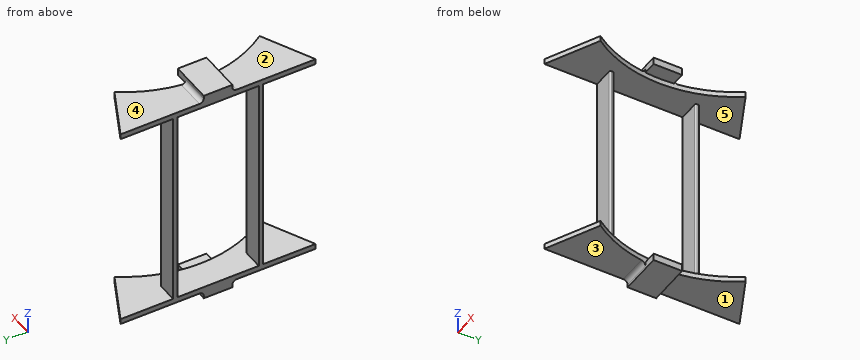
from build123d import *

# Parameters (mm, degrees)
BOSS_EXTRUDE1_DEPTH = 1.875
BOSS_EXTRUDE3_DEPTH = 140
BOSS_EXTRUDE4_DEPTH = 5
FILLET4_R           = 3


with BuildPart() as part:
    # Sketch1 → Boss-Extrude1 (new body, symmetric)
    with BuildSketch(Plane.XY):
        with BuildLine():
            Line((-72.585877034, -50.825178267), (-108.610994186, -68.325178267))
            Line((-108.610994186, -68.325178267), (-108.610994186, 68.325178267))
            Line((-108.610994186, 68.325178267), (-72.585877034, 50.825178267))
            ThreePointArc((-72.585877034, 50.825178267), (-88.610994186, 0), (-72.585877034, -50.825178267))
        make_face()
    boss_extrude1 = extrude(amount=BOSS_EXTRUDE1_DEPTH, both=True)

    # Sketch3 → Boss-Extrude3 (add)
    with BuildSketch(Plane.XY.offset(1.875)):
        with BuildLine():
            Line((-108.610994186, -28.5), (-108.610994186, -31.5))
            Line((-108.610994186, -31.5), (-94.610994186, -31.5))
            ThreePointArc((-94.610994186, -31.5), (-93.903887405, -31.207106781), (-93.610994186, -30.5))
            Line((-93.610994186, -30.5), (-93.610994186, -29.5))
            ThreePointArc((-93.610994186, -29.5), (-93.903887405, -28.792893219), (-94.610994186, -28.5))
            Line((-94.610994186, -28.5), (-108.610994186, -28.5))
        make_face()
    boss_extrude3 = extrude(amount=BOSS_EXTRUDE3_DEPTH)

    # Mirror2: Boss-Extrude3 across plane
    add(boss_extrude3.mirror(Plane.ZX))

    # Mirror7: Boss-Extrude1 across plane
    add(boss_extrude1.mirror(Plane.XY.offset(71.875)))

    # Sketch4 → Boss-Extrude4 (add)
    with BuildSketch(Plane(origin=(0, 0, -1.875), x_dir=(-1, 0, 0), z_dir=(0, 0, -1))):
        Polygon((108.610994186, 0), (108.610994186, 10), (78.610994186, 10), (78.610994186, -10), (108.610994186, -10), align=None)
    boss_extrude4 = extrude(amount=BOSS_EXTRUDE4_DEPTH)

    # Mirror10: Boss-Extrude4 across plane
    add(boss_extrude4.mirror(Plane.XY.offset(71.875)))

    # Fillet4
    fillet4_edges = [part.edges().sort_by_distance(p)[0] for p in [
        (-98.327958095, -10, -1.875),
        (-98.327958095, 10, -1.875),
        (-98.327958095, -10, 145.625),
        (-98.327958095, 10, 145.625),
    ]]
    fillet(fillet4_edges, radius=FILLET4_R)


solid = part.part
For this review, take the finished solid that the model builds, in its own axes (mm). Face numbers are marked on the shaded views. A direction names the side the tool comes from. Give positions to 0.01 mm unless a question says otherwise; leave off trailing zeros. Write each loop counter-clockwise with the first axis right and the second up, starting at its lowest first coordinate (ties: lowest second). Pieces come first, ordered by that corner, then holes. Notation, with made-up numbers: (75.5, 59) -> (125.5, 59) arc R18 cw to (125.5, 88) -> close; hole circle Ø11 at (32, 37.5). An arc over 180 degrees is marked (long way). Use CSV: the item, a comma, the result in double quotes.
Q1. Tool access review of the marked faces 1, 2 and 3: name each direction out of +Z, -Z, +X, -X, +Y, -Y from which nothing blocks a thin tool from reaching the whole face with its end or side.
Conclusion:
face 1,"-Z, +X, -X, +Y"
face 2,"+Z, +X, -X, -Y"
face 3,"-Z, +X, -X, -Y"
Q2. Take a section at D-D, the plane x = -98.5. Write out the cut boundary in (y, z) (3 decimals).
Conclusion:
outline,"(-63.414, -1.875) -> (-13, -1.875) arc R3 cw to (-10, -4.875) -> (-10, -6.875) -> (10, -6.875) -> (10, -4.875) arc R3 cw to (13, -1.875) -> (63.414, -1.875) -> (63.414, 1.875) -> (31.5, 1.875) -> (31.5, 141.875) -> (63.414, 141.875) -> (63.414, 145.625) -> (13, 145.625) arc R3 cw to (10, 148.625) -> (10, 150.625) -> (-10, 150.625) -> (-10, 148.625) arc R3 cw to (-13, 145.625) -> (-63.414, 145.625) -> (-63.414, 141.875) -> (-31.5, 141.875) -> (-31.5, 1.875) -> (-63.414, 1.875) -> close; hole (-28.5, 1.875) -> (28.5, 1.875) -> (28.5, 141.875) -> (-28.5, 141.875) -> close"
Q3. Take a section at A-A, the plane y = 0. Write out the cut boundary in (x, z) (3 decimals), then the cut area to 3 significant figures.
Conclusion:
outline,"(-108.611, -6.875) -> (-78.611, -6.875) -> (-78.611, -1.875) -> (-88.611, -1.875) -> (-88.611, 1.875) -> (-108.611, 1.875) -> close; (-108.611, 141.875) -> (-88.611, 141.875) -> (-88.611, 145.625) -> (-78.611, 145.625) -> (-78.611, 150.625) -> (-108.611, 150.625) -> close"
area,"450 mm2"
Q4. Mouldability with a two-part tool opening along Y and no side actions: class the marked faces 4 and 5 as pulls with the +Y half, pulls with the -Y half, needs draft (parallel to the pull), parting line crosses it, or undercut.
Conclusion:
face 4,"needs draft"
face 5,"undercut"
Q5. To check wall thickness, follow probe 1 along Z at (x, y) = (-95.5, -13.5) (3 decimals); probe 2 along Z at (x, y) = (-103, -2) (3 decimals); probe 3 along Y at (x, z) = (-105.5, 126). State the ranges of each line that lie inside material, in increasing order. Write a range as [from, to].
Conclusion:
probe 1,"[-1.875, 1.875], [141.875, 145.625]"
probe 2,"[-6.875, 1.875], [141.875, 150.625]"
probe 3,"[-31.5, -28.5], [28.5, 31.5]"
Q6. Take a section at B-B, the plane z = 79.5. Write out the cut boundary in (x, y), then the cut area to 3 significant figures.
Conclusion:
outline,"(-108.61, -31.5) -> (-94.61, -31.5) arc R1 ccw to (-93.61, -30.5) -> (-93.61, -29.5) arc R1 ccw to (-94.61, -28.5) -> (-108.61, -28.5) -> close; (-108.61, 28.5) -> (-94.61, 28.5) arc R1 ccw to (-93.61, 29.5) -> (-93.61, 30.5) arc R1 ccw to (-94.61, 31.5) -> (-108.61, 31.5) -> close"
area,"89.1 mm2"
Q7. For P1, Ø8, axis at x = -92.5, z = 110, coming from the -Y side; P2, Ø5, axis at y = -33.5, z = 115, coming from the +X side; P3, Ø5.5, axis at x = -86.5, z = 147, coming from the -Y side, all flat-tipped, find the tip position at first contact; note any pin that passes through.
Conclusion:
P1,"y = -31.5"
P2,"x = -93.74"
P3,"y = -58.74"
Q8. Take a section at C-C, the plane x = -82. Write out the cut boundary in (y, z) (3 decimals), then the cut area to 3 significant figures.
Conclusion:
outline,"(-55.398, -1.875) -> (-33.584, -1.875) -> (-33.584, 1.875) -> (-55.398, 1.875) -> close; (-55.398, 141.875) -> (-33.584, 141.875) -> (-33.584, 145.625) -> (-55.398, 145.625) -> close; (-10, -6.875) -> (10, -6.875) -> (10, -1.875) -> (-10, -1.875) -> close; (-10, 145.625) -> (10, 145.625) -> (10, 150.625) -> (-10, 150.625) -> close; (33.584, -1.875) -> (55.398, -1.875) -> (55.398, 1.875) -> (33.584, 1.875) -> close; (33.584, 141.875) -> (55.398, 141.875) -> (55.398, 145.625) -> (33.584, 145.625) -> close"
area,"527 mm2"
